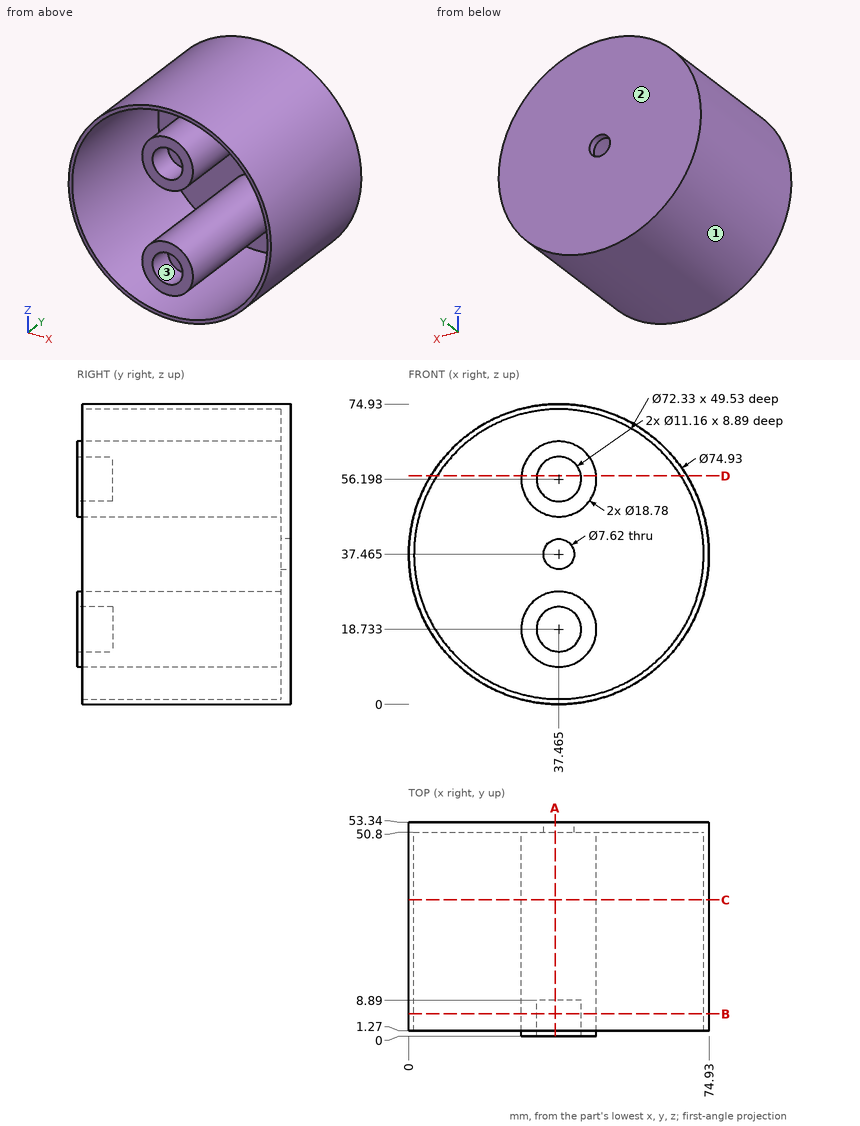
Verification items for this drawing (mm, ordinates from the low corner). Coordinates: 2 decimals unless noted, no trailing zeros. Order: outer loops, then holes, each group sorted by start corner. A loop starts at its lowest first (then second) coordinate and runs counter-clockwise, first axis right, second up. Notation, with made-up numbers: M -9.75,-29.75 L 3.25,-29.75 A17 cw 3.25,-3.75 Z; hole C -39,-5 d11. An arc over 180 degrees is marked long. One line per item, written item: value. Start each with the question number.
Item 1: Thickness scan on probe 1 along X at (y, z) = (16, 23.5) (1 decimal); probe 2 along X at (y, z) = (43.5, 54.5) (1 decimal); probe 3 along X at (y, z) = (24, 36.5). Record the ranges inside material, lowest first.
Item 2: Mould release check, pull along X, two halves, no side actions. Record for the marked faces 1, 2 and 3: pulls with the +X half, pulls with the -X half, needs draft (parallel to the pull), parting line crosses it, or undercut.
Item 3: Sectioned sample at C-C on y = 34. Record the cut outline in (x, z) (1 decimal).
Item 4: Sectioned sample at A-A on x = 36.5. Record the cut outline in (y, z), then the cut area to 3 significant figures.
Item 5: Sectioned sample at B-B on y = 5.5. Record the cut outline in (x, z) (1 decimal).
Item 6: Depth check by flat-ended pin: P1, Ø1, axis at x = 42.5, y = 8.5, coming from the -Z side (1 decimal); P2, Ø5, axis at x = 23.5, y = 31, coming from the +Z side; P3, Ø1, axis at x = 55.5, z = 8, coming from the -Y side. Enter the tip coordinate at first touch or a pass-through.
Item 7: Sectioned sample at D-D on z = 57. Record the cut outline in (x, y), then the cut area to 3 significant figures.
Calculated:
1. probe 1: 2.7 to 4.1, 29.4 to 45.6, 70.8 to 72.2
1. probe 2: 4.1 to 5.6, 28.2 to 46.7, 69.4 to 70.8
1. probe 3: 0.01 to 1.31, 73.62 to 74.92
2. face 1: parting line crosses it
2. face 2: needs draft
2. face 3: undercut
3. outline: C 37.5,37.5 d74.9; C 37.5,18.7 d18.8; C 37.5,56.2 d18.8; hole C 37.5,37.5 d72.3
4. outline: M 0,9.39 L 50.8,9.39 L 50.8,1.31 L 1.27,1.31 L 1.27,0.01 L 53.34,0.01 L 53.34,33.78 L 50.8,33.78 L 50.8,28.07 L 0,28.07 L 0,24.23 L 8.89,24.23 L 8.89,13.24 L 0,13.24 Z; M 0,46.86 L 50.8,46.86 L 50.8,41.15 L 53.34,41.15 L 53.34,74.92 L 1.27,74.92 L 1.27,73.62 L 50.8,73.62 L 50.8,65.54 L 0,65.54 L 0,61.69 L 8.89,61.69 L 8.89,50.7 L 0,50.7 Z
4. area: 2,000 mm^2
5. outline: C 37.5,37.5 d74.9; C 37.5,18.7 d18.8; C 37.5,56.2 d18.8; hole C 37.5,37.5 d72.3; hole C 37.5,18.7 d11.2; hole C 37.5,56.2 d11.2
6. P1: z = 0.3
6. P2: z = 73.13
6. P3: y = 50.8
7. outline: M 5.5,1.27 L 7.03,1.27 L 7.03,50.8 L 28.11,50.8 L 28.11,0 L 31.94,0 L 31.94,8.89 L 42.99,8.89 L 42.99,0 L 46.82,0 L 46.82,50.8 L 67.9,50.8 L 67.9,1.27 L 69.43,1.27 L 69.43,53.34 L 5.5,53.34 Z
7. area: 1,170 mm^2
